```python
from build123d import *

# Parameters (mm, degrees)
SKETCH1_W                       = 150
SKETCH1_H                       = 124
BOSS_EXTRUDE1_DEPTH             = 87.5
BOSS_EXTRUDE2_REACH             = 132.863
SKETCH8_W                       = 210
SKETCH8_H                       = 20
BOSS_EXTRUDE2_DIRECTION_2_REACH = 132.863
CUT_EXTRUDE1_REACH              = 221.941
SKETCH2_R                       = 41
M10_TAPPED_HOLE1_D              = 8.5
M10_TAPPED_HOLE1_DEPTH          = 27.5
M10_TAPPED_HOLE1_TIP            = 2.553657631
FILLET1_R                       = 10
CHAMFER1_SIZE                   = 5
CHAMFER2_SIZE                   = 1


with BuildPart() as part:
    # Sketch1 → Boss-Extrude1 (new, symmetric)
    with BuildSketch(Plane.XY):
        Rectangle(SKETCH1_W, SKETCH1_H)
    extrude(amount=BOSS_EXTRUDE1_DEPTH, both=True)

    # Boss-Extrude2: up to this face of the body (flat: up to its plane)
    boss_extrude2_end = Plane(part.part.faces().sort_by_distance((0, 0, -87.5))[0])
    # Sketch8 → Boss-Extrude2 (add, up to the picked face)
    with BuildSketch(Plane.XY, mode=Mode.PRIVATE) as boss_extrude2_sk1:
        with Locations((0, 72)):
            Rectangle(SKETCH8_W, SKETCH8_H)
    boss_extrude2_tool1 = split(extrude(boss_extrude2_sk1.sketch, amount=-BOSS_EXTRUDE2_REACH, mode=Mode.PRIVATE), bisect_by=boss_extrude2_end, keep=Keep.BOTH, mode=Mode.PRIVATE)
    add(boss_extrude2_tool1.solids().sort_by(Axis((0, 72, 0), (0, 0, -1)))[0])

    # Boss-Extrude2 direction 2: up to this face of the body (flat: up to its plane)
    boss_extrude2_direction_2_end = Plane(part.part.faces().sort_by_distance((0, 0, 87.5))[0])
    # Sketch8 → Boss-Extrude2 direction 2 (add, up to the picked face)
    with BuildSketch(Plane.XY, mode=Mode.PRIVATE) as boss_extrude2_direction_2_sk1:
        with Locations((0, 72)):
            Rectangle(SKETCH8_W, SKETCH8_H)
    boss_extrude2_direction_2_tool1 = split(extrude(boss_extrude2_direction_2_sk1.sketch, amount=BOSS_EXTRUDE2_DIRECTION_2_REACH, mode=Mode.PRIVATE), bisect_by=boss_extrude2_direction_2_end, keep=Keep.BOTH, mode=Mode.PRIVATE)
    add(boss_extrude2_direction_2_tool1.solids().sort_by(Axis((0, 72, 0), (0, 0, 1)))[0])

    # Sketch2 → Cut-Extrude1 (cut, up to next)
    with BuildSketch(Plane.XY.offset(87.5), mode=Mode.PRIVATE) as cut_extrude1_sk1:
        Circle(SKETCH2_R)
    cut_extrude1_tool1 = extrude(cut_extrude1_sk1.sketch, amount=-CUT_EXTRUDE1_REACH, mode=Mode.PRIVATE) & part.part
    add(cut_extrude1_tool1.solids().sort_by_distance((0, 0, 87.5))[0], mode=Mode.SUBTRACT)

    # M10 Tapped Hole1
    with Locations(Plane.XY.offset(87.5)):
        with Locations((-36.062445841, -36.062445841), (-36.062445841, 36.062445841), (-51, 0), (36.062445841, 36.062445841), (51, 0), (36.062445841, -36.062445841)):
            Hole(M10_TAPPED_HOLE1_D / 2, depth=M10_TAPPED_HOLE1_DEPTH)
            with Locations((0, 0, -(M10_TAPPED_HOLE1_DEPTH + M10_TAPPED_HOLE1_TIP / 2))):  # 118° drill point
                Cone(0, M10_TAPPED_HOLE1_D / 2, M10_TAPPED_HOLE1_TIP, mode=Mode.SUBTRACT)

    # Fillet1
    fillet1_edges = [part.edges().sort_by_distance(p)[0] for p in [
        (-75, 62, 0),
        (75, 62, 0),
    ]]
    fillet(fillet1_edges, radius=FILLET1_R)

    # Chamfer1
    chamfer1_edges = [part.edges().sort_by_distance(p)[0] for p in [
        (-95, 62, -87.5),
        (95, 62, 87.5),
        (105, 62, 0),
        (105, 72, -87.5),
        (105, 82, 0),
        (105, 72, 87.5),
        (0, 82, -87.5),
        (-105, 82, 0),
        (0, 82, 87.5),
        (-105, 72, -87.5),
        (-105, 62, 0),
        (-105, 72, 87.5),
        (0, -62, 87.5),
        (75, -5, 87.5),
        (0, -62, -87.5),
        (75, -5, -87.5),
        (-75, -5, -87.5),
        (-75, -5, 87.5),
        (-95, 62, 87.5),
        (95, 62, -87.5),
        (-77.928932188, 59.071067812, -87.5),
        (-77.928932188, 59.071067812, 87.5),
        (77.928932188, 59.071067812, -87.5),
        (77.928932188, 59.071067812, 87.5),
        (75, -62, 0),
        (-75, -62, 0),
    ]]
    chamfer(chamfer1_edges, length=CHAMFER1_SIZE)

    # Chamfer2
    chamfer2_edges = [part.edges().sort_by_distance(p)[0] for p in [
        (-41, 0, -87.5),
        (-41, 0, 87.5),
        (-31.812445841, -36.062445841, 87.5),
        (-46.75, 0, 87.5),
        (-31.812445841, 36.062445841, 87.5),
        (40.312445841, -36.062445841, 87.5),
        (55.25, 0, 87.5),
        (40.312445841, 36.062445841, 87.5),
    ]]
    chamfer(chamfer2_edges, length=CHAMFER2_SIZE)


solid = part.part
```
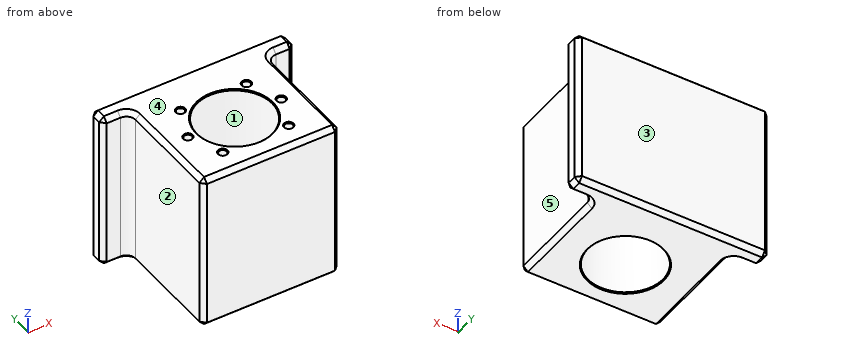
Input: part model. Units: mm. Frame: model coordinates. Face numbers are marked on the shaded views. A direction names the side the tool comes from. Coordinates: 2 decimals unless noted, no trailing zeros. Write each loop counter-clockwise with the first axis right and the second up, starting at its lowest first coordinate (ties: lowest second). Pieces come first, ordered by that corner, then holes.
1) Mould query, pull axis Y, two halves, no side actions, for the marked faces 1, 2 and 3. Classes: pulls with the +Y half, pulls with the -Y half, needs draft (parallel to the pull), parting line crosses it, or undercut.
2) Set-up query: the marked faces 4 and 5. Return all of +Z, -Z, +X, -X, +Y, -Y with unobstructed straight access to the full face (end or side cutting, diameter ignored); none if empty.
3) Material intervals for line 1 along Y through (x, z) = (51, 75.75); line 2 along X through (y, z) = (-7.5, -53); line 3 along Y through (x, z) = (25, 30), sorted ascending.
4) Section B-B on z = 39. Output: boundary loops of the cut face in (x, y).
5) Section C-C on y = 48. Output: boundary loops of the cut face in (x, z).
6) Section A-A on x = 0. Output: boundary loops of the cut face in (y, z), and give its area (3 significant figures).
7) Pin query (flat end, axial travel): pin 1 Ø1 at (y, z) = (-17, 47) entering from -X; pin 2 Ø3 at (y, z) = (-22.5, -65.5) entering from +X; pin 3 Ø4.5 at (x, z) = (-91.5, 38) entering from -Y. Return the tip coordinate at first contact, or that it passes through.
Check result:
1. face 1: undercut
1. face 2: needs draft
1. face 3: pulls with the +Y half
2. face 4: +Z, +X, -X, +Y, -Y
2. face 5: +Z, -Z, +X, -Y
3. line 1: y = -62 to -4.25, 4.25 to 82
3. line 2: x = -75 to -40.31, 40.31 to 75
3. line 3: y = -62 to -32.5, 32.5 to 82
4. outline: (-105, 67) - (-100, 62) - (-85, 62) arc R10 cw to (-75, 52) - (-75, -57) - (-70, -62) - (70, -62) - (75, -57) - (75, 52) arc R10 cw to (85, 62) - (100, 62) - (105, 67) - (105, 77) - (100, 82) - (-100, 82) - (-105, 77) - close; hole circle Ø82 at (0, 0)
5. outline: (-75, -82.5) - (-70, -87.5) - (70, -87.5) - (75, -82.5) - (75, 82.5) - (70, 87.5) - (-70, 87.5) - (-75, 82.5) - close
6. outline: (-62, -82.5) - (-57, -87.5) - (-42, -87.5) - (-41, -86.5) - (-41, 86.5) - (-42, 87.5) - (-57, 87.5) - (-62, 82.5) - close; (41, -86.5) - (42, -87.5) - (77, -87.5) - (82, -82.5) - (82, 82.5) - (77, 87.5) - (42, 87.5) - (41, 86.5) - close
6. area: 10,800 mm2
7. pin 1: stops at x = -75
7. pin 2: stops at x = 75
7. pin 3: stops at y = 62
